Input: part model. Units: mm. Frame: model coordinates. Round coordinates to 2 decimals unless told otherwise and drop trailing zeros. Write each loop counter-clockwise with the first axis right and the second up, starting at its lowest first coordinate (ties: lowest second). Pieces come first, ordered by that corner, then holes. Notation, with made-up numbers: (57.25, 31) - (83.25, 31) arc R28 ccw to (83.25, 54) - close; hole circle Ø3 at (62.25, 38.25). An arc over 180 degrees is marked (long way). Use one line per item in the form item = value.
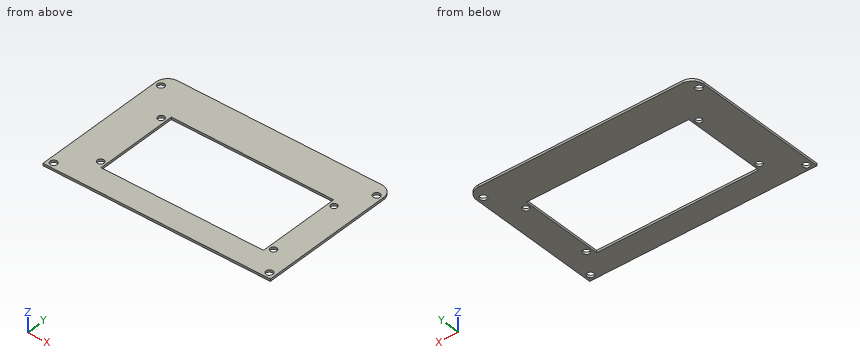
Autodesk Inventor part; units mm, degrees
ref_plane "YZ Plane" through (0, 0, 0) normal (1, 0, 0) x (0, 1, 0)
ref_plane "XZ Plane" through (0, 0, 0) normal (0, 1, 0) x (-1, 0, 0)
ref_plane "XY Plane" through (0, 0, 0) normal (0, 0, 1) x (1, 0, 0)
ref_plane "Work Plane1" through (0, 0, 0) normal (0, 0, 1) x (1, 0, 0)
sketch "Sketch1" plane through (0, 0, 0) normal (0, 0, 1) x (1, 0, 0)
  circle A0 centre (2.5, -2.5) radius 1.5
  circle A1 centre (95.5, -57.5) radius 1.5
  circle A2 centre (95.5, -2.5) radius 1.5
  circle A3 centre (2.5, -57.5) radius 1.5
  line L0 (50.7939, -5.85) -> (93.3881, -5.85)
  line L1 (93.3881, -5.85) -> (93.3881, -53.8601)
  line L2 (93.3881, -53.8601) -> (4, -53.8601)
  line L3 (4, -53.8601) -> (4, -5.85)
  line L4 (4, -5.85) -> (5.9071, -5.85)
  line L5 (5.9071, -5.85) -> (5.9071, 0)
  line L6 (5.9071, 0) -> (50.7939, 0)
  line L7 (50.7939, 0) -> (50.7939, -5.85)
  line L8 (98, 3) -> (98, -60)
  line L9 (0, 3) -> (98, 3)
  line L10 (0, -60) -> (0, 3)
  line L11 (0, -60) -> (98, -60)
  line L12 (16.205, -49.4986) -> (86.205, -49.4986)
  line L13 (86.205, -49.4986) -> (86.205, -13.4986)
  line L14 (86.205, -13.4986) -> (16.205, -13.4986)
  line L15 (16.205, -13.4986) -> (16.205, -49.4986)
  line L16 (88.455, -46.9986) -> (13.955, -46.9986) construction
  line L17 (13.955, -46.9986) -> (13.955, -15.9986) construction
  line L18 (13.955, -15.9986) -> (88.455, -15.9986) construction
  line L19 (88.455, -15.9986) -> (88.455, -46.9986) construction
  line L20 (88.455, -46.9986) -> (13.955, -15.9986) construction
  line L21 (13.955, -46.9986) -> (88.455, -15.9986) construction
  circle A4 centre (13.955, -15.9986) radius 1.4
  circle A5 centre (13.955, -46.9986) radius 1.4
  circle A6 centre (88.455, -15.9986) radius 1.4 construction
  circle A7 centre (88.455, -46.9986) radius 1.4
  circle A8 centre (88.455, -15.9986) radius 1.4
  point P0 (0, 0)
  point P1 (51.205, -31.4986)
  dimension "d0" = 70
  dimension "d1" = 36
  dimension "d2" = 74.5
  dimension "d3" = 31
  dimension "d4" = 2.8
  dimension "d5" = 2.8
  dimension "d6" = 2.8
  dimension "d7" = 2.8
extrude "Extrusion1" add sketch "Sketch1" along normal blind 1 contours L0 L1 L2 L3 L4 L5 L6 L7 | L8 L11 L10 L9
fillet "Fillet1" radius 5 2 edges at (98, 3, 0.5) (0, 3, 0.5)
sketch "Sketch2" plane through (0, 0, 1) normal (0, 0, 1) x (1, 0, 0)
  arc A0 (5, 3) -> (0, -2) centre (5, -2) ccw
  line L0 (0, -2) -> (0, -60)
  line L1 (0, -60) -> (98, -60)
  line L2 (98, -60) -> (98, -2)
  arc A1 (98, -2) -> (93, 3) centre (93, -2) ccw
  line L3 (93, 3) -> (5, 3)
  line L4 (16.205, -49.4986) -> (16.205, -13.4986)
  line L5 (16.205, -13.4986) -> (86.205, -13.4986)
  line L6 (86.205, -13.4986) -> (86.205, -49.4986)
  line L7 (86.205, -49.4986) -> (16.205, -49.4986)
  circle A2 centre (88.455, -15.9986) radius 1.4
  circle A3 centre (88.455, -46.9986) radius 1.4
  circle A4 centre (13.955, -46.9986) radius 1.4
  circle A5 centre (13.955, -15.9986) radius 1.4
  circle A6 centre (2.5, -57.5) radius 1.5
  circle A7 centre (95.5, -2.5) radius 1.5
  circle A8 centre (95.5, -57.5) radius 1.5
  circle A9 centre (2.5, -2.5) radius 1.5
  line L8 (9.9881, -3.9779) -> (87.4866, -3.9779) construction
  line L9 (87.4866, -3.9779) -> (87.4866, -10.4067) construction
  line L10 (87.4866, -10.4067) -> (9.9881, -10.4067) construction
  line L11 (9.9881, -10.4067) -> (9.9881, -3.9779) construction
  point P0 (0, 0)
properties part number "04_Adapterplate_Display"
(1) First-contact query: pin 1 Ø1.8 at (x, y) = (2.5, -2.5) entering from +Z (1 decimal). Flat tip, straight axial feed; report the tip coordinate or a pass-through.
Derived:
pin_1 = through
(2) Cut plane A-A on y = -29.5. Output: boundary loops of the cut face in (x, z) (3 decimals), then the cut area to 3 significant figures.
Derived:
outline = (0, 0) - (16.205, 0) - (16.205, 1) - (0, 1) - close; (86.205, 0) - (98, 0) - (98, 1) - (86.205, 1) - close
area = 28.0 mm^2
(3) Cut plane B-B on x = 24. Output: boundary loops of the cut face in (y, z), then the cut area to 3 significant figures.
Derived:
outline = (-60, 0) - (-49.5, 0) - (-49.5, 1) - (-60, 1) - close; (-13.5, 0) - (3, 0) - (3, 1) - (-13.5, 1) - close
area = 27.0 mm^2
(4) Material intervals for L1, parallel to X at y = -30, z = 0.4 (3 decimals); L2, parallel to Y at x = 56.5, z = 0.1; L3, parallel to X at y = -15, z = 0.95 (3 decimals), sorted ascending.
Derived:
L1 = 0 to 16.205, 86.205 to 98
L2 = -60 to -49.5, -13.5 to 3
L3 = 0 to 12.974, 14.936 to 16.205, 86.205 to 87.474, 89.436 to 98
(5) Cut plane C-C on z = 0.3. Count the separate pieces of the cut face and the enclosed holes in it, then the cut area to 3 significant figures.
Derived:
separate_pieces = 1
enclosed_holes = 9
area = 3,590 mm^2
(6) Cut plane D-D on x = 95.5. Output: boundary loops of the cut face in (y, z).
Derived:
outline = (-60, 0) - (-59, 0) - (-59, 1) - (-60, 1) - close; (-56, 0) - (-4, 0) - (-4, 1) - (-56, 1) - close; (-1, 0) - (2.33, 0) - (2.33, 1) - (-1, 1) - close
